```python
from build123d import *

# Parameters (mm, degrees)
F1_DEPTH = 3


with BuildPart() as f1:
    # F0 (on Front) → F1 (new body)
    with BuildSketch(Plane.XZ):
        with BuildLine():
            ThreePointArc((-55, -36), (-53.828427, -38.828427), (-51, -40))
            Line((-51, -40), (39.171573, -40))
            ThreePointArc((39.171573, -40), (39.93694, -39.847759), (40.585786, -39.414214))
            Line((40.585786, -39.414214), (53.828427, -26.171573))
            ThreePointArc((53.828427, -26.171573), (54.695518, -24.873879), (55, -23.343146))
            Line((55, -23.343146), (55, -13.837789))
            ThreePointArc((55, -13.837789), (55.267949, -12.837789), (56, -12.105738))
            Line((56, -12.105738), (64.93, -6.95))
            Line((64.93, -6.95), (64.93, -4.95))
            Line((64.93, -4.95), (61.93, -4.95))
            Line((61.93, -4.95), (61.93, 4.95))
            Line((61.93, 4.95), (64.93, 4.95))
            Line((64.93, 4.95), (64.93, 6.95))
            Line((64.93, 6.95), (56, 12.105738))
            ThreePointArc((56, 12.105738), (55.267949, 12.837789), (55, 13.837789))
            Line((55, 13.837789), (55, 23.343146))
            ThreePointArc((55, 23.343146), (54.695518, 24.873879), (53.828427, 26.171573))
            Line((53.828427, 26.171573), (40.585786, 39.414214))
            ThreePointArc((40.585786, 39.414214), (39.93694, 39.847759), (39.171573, 40))
            Line((39.171573, 40), (35.757359, 40))
            Line((35.757359, 40), (-51, 40))
            ThreePointArc((-51, 40), (-53.828427, 38.828427), (-55, 36))
            Line((-55, 36), (-55, -36))
        make_face()
        with BuildLine():
            ThreePointArc((-47, -37), (-50.535534, -35.535534), (-52, -32))
            Line((-52, -32), (-52, -3.732051))
            ThreePointArc((-52, -3.732051), (-51.258819, -2.766125), (-50.133975, -3.232051))
            Line((-50.133975, -3.232051), (-31.504065, -35.5))
            ThreePointArc((-31.504065, -35.5), (-31.504065, -36.5), (-32.370091, -37))
            Line((-32.370091, -37), (-47, -37))
        make_face(mode=Mode.SUBTRACT)
        with BuildLine():
            Line((-28.905989, -36), (-51.732051, 3.535898))
            ThreePointArc((-51.732051, 3.535898), (-51.931852, 4.01826), (-52, 4.535898))
            Line((-52, 4.535898), (-52, 33.282309))
            ThreePointArc((-52, 33.282309), (-50.665874, 35.020975), (-48.641154, 34.182309))
            Line((-48.641154, 34.182309), (-8.410055, -35.5))
            ThreePointArc((-8.410055, -35.5), (-8.410055, -36.5), (-9.27608, -37))
            Line((-9.27608, -37), (-27.173938, -37))
            ThreePointArc((-27.173938, -37), (-28.173938, -36.732051), (-28.905989, -36))
        make_face(mode=Mode.SUBTRACT)
        with BuildLine():
            ThreePointArc((-46.226497, 34), (-46.226497, 36), (-44.494447, 37))
            Line((-44.494447, 37), (-28.328639, 37))
            ThreePointArc((-28.328639, 37), (-27.328639, 36.732051), (-26.596588, 36))
            Line((-26.596588, 36), (14.683956, -35.5))
            ThreePointArc((14.683956, -35.5), (14.683956, -36.5), (13.817931, -37))
            Line((13.817931, -37), (-4.079928, -37))
            ThreePointArc((-4.079928, -37), (-5.079928, -36.732051), (-5.811978, -36))
            Line((-5.811978, -36), (-46.226497, 34))
        make_face(mode=Mode.SUBTRACT)
        with BuildLine():
            Line((17.282032, -36), (-23.998512, 35.5))
            ThreePointArc((-23.998512, 35.5), (-23.998512, 36.5), (-23.132487, 37))
            Line((-23.132487, 37), (-5.234628, 37))
            ThreePointArc((-5.234628, 37), (-4.234628, 36.732051), (-3.502577, 36))
            Line((-3.502577, 36), (36.911941, -34))
            ThreePointArc((36.911941, -34), (36.911941, -36), (35.179891, -37))
            Line((35.179891, -37), (19.014083, -37))
            ThreePointArc((19.014083, -37), (18.014083, -36.732051), (17.282032, -36))
        make_face(mode=Mode.SUBTRACT)
        with BuildLine():
            Line((52, -20.669182), (52, -22.100505))
            ThreePointArc((52, -22.100505), (51.695518, -23.631239), (50.828427, -24.928932))
            Line((50.828427, -24.928932), (41.992628, -33.764731))
            ThreePointArc((41.992628, -33.764731), (40.317362, -34.333407), (38.846364, -33.350518))
            Line((38.846364, -33.350518), (-0.904501, 35.5))
            ThreePointArc((-0.904501, 35.5), (-0.904501, 36.5), (-0.038476, 37))
            Line((-0.038476, 37), (18.436733, 37))
            ThreePointArc((18.436733, 37), (18.936733, 36.866025), (19.302758, 36.5))
            Line((19.302758, 36.5), (51.732051, -19.669182))
            ThreePointArc((51.732051, -19.669182), (51.931852, -20.151544), (52, -20.669182))
        make_face(mode=Mode.SUBTRACT)
        with BuildLine():
            Line((50.133975, -12.901233), (23.055535, 34))
            ThreePointArc((23.055535, 34), (23.055535, 36), (24.787586, 37))
            Line((24.787586, 37), (37.928932, 37))
            ThreePointArc((37.928932, 37), (38.694299, 36.847759), (39.343146, 36.414214))
            Line((39.343146, 36.414214), (50.828427, 24.928932))
            ThreePointArc((50.828427, 24.928932), (51.695518, 23.631239), (52, 22.100505))
            Line((52, 22.100505), (52, -12.401233))
            ThreePointArc((52, -12.401233), (51.258819, -13.367159), (50.133975, -12.901233))
        make_face(mode=Mode.SUBTRACT)
    extrude(amount=F1_DEPTH)


solid = f1.part
```
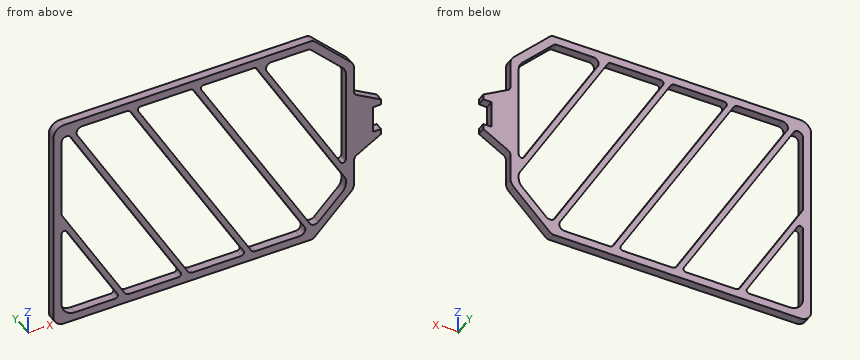
CAD build for the part. Positions are in the model's coordinates, mm. Coordinates: 2 decimals unless noted, no trailing zeros. Write each loop counter-clockwise with the first axis right and the second up, starting at its lowest first coordinate (ties: lowest second). Pieces come first, ordered by that corner, then holes. Notation, with made-up numbers: (73, 31) -> (101, 31) arc R25 ccw to (101, 50) -> close; hole circle Ø10 at (-17, -1.75). An arc over 180 degrees is marked (long way). Use CSV: the item, a comma, the result in double quotes. Start each with the question number.
Item 1: Band-saw the part on D-D, the plane y = -2. Give the number of separate pieces and of enclosed holes in the cut face, plus the area to 3 significant figures.
Item 2: Band-saw the part on C-C, the plane x = -15. Write the cut outline in (y, z).
Item 3: Drop flat-ended pins along their axis: P1, Ø1.5, axis at y = -2, z = -12.5, coming from the +X side; P2, Ø0.9, axis at y = -2, z = -20.5, coming from the +X side; P3, Ø1.5, axis at y = -2, z = -2, coming from the +X side. Give the stop position or say it passes through.
Item 4: Band-saw the part on A-A, the plane z = -15. Write the cut outline in (x, y).
Item 5: Band-saw the part on B-B, the plane x = 48. Write the cut outline in (y, z).
Item 6: Wall check: probe 1 along X at (y, z) = (-1.2, 4.5); probe 2 along Z at (x, y) = (33, -2.5); probe 3 along Z at (x, y) = (3.5, -2.75). Give the ranges that are in metal, low to high.
Response values:
1,separate pieces,"1"
1,enclosed holes,"6"
1,area,"1,970 mm2"
2,outline,"(-3, -40) -> (0, -40) -> (0, -37) -> (-3, -37) -> close; (-3, -24.09) -> (0, -24.09) -> (0, -20.09) -> (-3, -20.09) -> close; (-3, 15.91) -> (0, 15.91) -> (0, 19.91) -> (-3, 19.91) -> close; (-3, 37) -> (0, 37) -> (0, 40) -> (-3, 40) -> close"
3,P1,"stops at x = 56.62"
3,P2,"stops at x = 55"
3,P3,"stops at x = 61.93"
4,outline,"(-55, -3) -> (-52, -3) -> (-52, 0) -> (-55, 0) -> close; (-43.34, -3) -> (-41.03, -3) -> (-41.03, 0) -> (-43.34, 0) -> close; (-20.25, -3) -> (-17.94, -3) -> (-17.94, 0) -> (-20.25, 0) -> close; (2.85, -3) -> (5.16, -3) -> (5.16, 0) -> (2.85, 0) -> close; (25.94, -3) -> (28.25, -3) -> (28.25, 0) -> (25.94, 0) -> close; (49.04, -3) -> (55, -3) -> (55, 0) -> (49.04, 0) -> close"
5,outline,"(-3, -32) -> (0, -32) -> (0, -27.76) -> (-3, -27.76) -> close; (-3, -13.21) -> (0, -13.21) -> (0, -9.21) -> (-3, -9.21) -> close; (-3, 27.76) -> (0, 27.76) -> (0, 32) -> (-3, 32) -> close"
6,probe 1,"x = -55 to -52, -31.5 to -29.19, -8.41 to -6.1, 14.68 to 16.99, 37.78 to 40.09, 52 to 61.93"
6,probe 2,"z = -40 to -37, -27.22 to -23.22, 12.78 to 16.78, 37 to 40"
6,probe 3,"z = -40 to -37, -16.13 to -12.13, 23.87 to 27.87, 37 to 40"
